Input: part model. Units: mm. Frame: model coordinates. A direction names the side the tool comes from. Coordinates: 2 decimals unless noted, no trailing zeros. Loops run counter-clockwise (first coordinate to the right, second up) from the corner with the lowest first, then second, coordinate; pieces in that order, holes last.
Item 1: Contact query for flat-ended pins moving along their axis: P1, Ø12, axis at x = -10.5, z = 0.5, coming from the -Y side; P2, Ø3, axis at x = -42.5, z = 0, coming from the +Y side; P3, Ø3, axis at x = 11.5, z = -12, coming from the +Y side. Output: stop coordinate, or through.
Item 2: Section B-B on y = 0.45. Return loops of the section in (x, z).
Item 3: Pull-direction query (Z, two-part tool) for faces 3 (the cylindrical face through (-47.01, 0.79, 0.1)), 4 (the cylindrical face through (-1.673, 1.354, -0.074)), 5 (the cylindrical face through (-35.32, 0.79, -9.96)); classes: released by +Z, released by -Z, zero draft, split by the parting line, or undercut.
Item 4: Section C-C on x = -0.5. Return loops of the section in (y, z), and give its area (3 significant figures).
Item 5: Ray query, line 1 along Z through (x, y) = (0, 1.4) (3 decimals); line 2 along X through (y, z) = (1.4, -38.1); line 3 along Z through (x, y) = (-42.5, 1.05). Return the intervals inside material, ascending.
Item 6: Reachability of faces 1 (the flat face through (-13, 1.1, 12)), 2 (the cylindrical face through (-40.502, 0.789, -0.088)) from +Z, -Z, +X, -X, +Y, -Y: full face, straight path, thin tool, end or side. Return the list, or none.
Item 7: Section D-D on z = 28. Return loops of the section in (x, y).
Item 8: Section A-A on z = 0. Return loops of the section in (x, y) (1 decimal).
Autodesk Inventor part; units mm, degrees
ref_plane "YZ Plane" through (0, 0, 0) normal (1, 0, 0) x (0, 1, 0)
ref_plane "XZ Plane" through (0, 0, 0) normal (0, 1, 0) x (-1, 0, 0)
ref_plane "XY Plane" through (0, 0, 0) normal (0, 0, 1) x (1, 0, 0)
sketch "Sketch1" plane through (0, 0, 0) normal (0, 1, 0) x (-1, 0, 0)
  circle A0 centre (42.5, 0) radius 2
  circle A1 centre (-21.25, 36.8061) radius 2
  circle A2 centre (-21.25, -36.8061) radius 2
  line L0 (-21.25, -36.8061) -> (0, 0) construction
  arc A3 (-25.1562, -34.5508) -> (-20.8492, -41.2987) centre (-21.25, -36.8061) ccw
  line L1 (-21.25, 36.8061) -> (0, 0) construction
  arc A4 (-17.3438, 39.0613) -> (-25.1562, 34.5508) centre (-21.25, 36.8061) ccw
  line L2 (0, 0) -> (42.5, 0) construction
  arc A5 (42.5, -4.5105) -> (42.5, 4.5105) centre (42.5, 0) ccw
  line L3 (-21.6508, -41.2987) -> (28.2014, -41.2987)
  line L4 (28.2014, -41.2987) -> (33.3458, -35.9407)
  line L5 (33.3458, -35.9407) -> (33.3458, -15.3261)
  line L6 (-25.1562, -34.5508) -> (-22.1167, -29.2863)
  line L7 (36.421, -4.5105) -> (42.5, -4.5105)
  line L8 (42.5, 0) -> (36.6992, 0)
  line L9 (4.5105, 0) -> (0, 0)
  line L10 (42.5, 4.5105) -> (36.421, 4.5105)
  line L11 (-25.1562, 34.5508) -> (-22.1167, 29.2863)
  line L12 (-14.3043, 33.7968) -> (-17.3438, 39.0613)
  arc A6 (-22.1167, 29.2863) -> (-22.1167, -29.2863) centre (0, 0) ccw
  arc A7 (33.3458, -15.3261) -> (36.421, -4.5105) centre (0, 0) ccw
  arc A8 (36.421, 4.5105) -> (-14.3043, 33.7968) centre (0, 0) ccw
  point P0 (-10.625, -18.403)
  point P1 (-10.625, 18.403)
  point P2 (21.25, 0)
  dimension "d1" = 4
  dimension "d2" = 42.5
  dimension "d5" = 360
extrude "Extrusion1" add sketch "Sketch1" along normal blind 1.6 contours L6 A6 L11 A4 L12 A8 L10 A5 L7 A7 L5 L4 L3 A3
sketch "Sketch2" plane through (0, 1.6, 0) normal (0, 1, 0) x (1, 0, 0)
  line L0 (35, 0) -> (0, 0) construction
  circle A0 centre (12.5, 12.5) radius 3
  circle A1 centre (-12.5, 12.5) radius 3
  circle A2 centre (-12.5, -12.5) radius 3
  circle A3 centre (12.5, -12.5) radius 3
  line L1 (1.675, -1.675) -> (-1.675, -1.675)
  line L2 (-1.675, -1.675) -> (-1.675, 1.675)
  line L3 (-1.675, 1.675) -> (1.675, 1.675)
  line L4 (1.675, 1.675) -> (1.675, -1.675)
  line L5 (1.675, -1.675) -> (-1.675, 1.675) construction
  line L6 (-1.675, -1.675) -> (1.675, 1.675) construction
  circle A4 centre (0, 0) radius 1.675
  circle A5 centre (0, -28) radius 3.75
  line L7 (0, -28) -> (0, 0) construction
  line L8 (-42.5, -4.5105) -> (-36.421, -4.5105)
  arc A6 (-42.5, 4.5105) -> (-42.5, -4.5105) centre (-42.5, 0) ccw
  line L9 (-36.421, 4.5105) -> (-42.5, 4.5105)
  arc A7 (-33.3458, 15.3261) -> (-36.421, 4.5105) centre (0, 0) ccw
  line L10 (-33.3458, 35.9407) -> (-33.3458, 15.3261)
  line L11 (-28.2014, 41.2987) -> (-33.3458, 35.9407)
  line L12 (21.6508, 41.2987) -> (-28.2014, 41.2987)
  arc A8 (25.1562, 34.5508) -> (21.6508, 41.2987) centre (21.25, 36.8061) ccw
  line L13 (22.1167, 29.2863) -> (25.1562, 34.5508)
  arc A9 (22.1167, -29.2863) -> (22.1167, 29.2863) centre (0, 0) ccw
  line L14 (25.1562, -34.5508) -> (22.1167, -29.2863)
  arc A10 (17.3438, -39.0613) -> (25.1562, -34.5508) centre (21.25, -36.8061) ccw
  line L15 (14.3043, -33.7968) -> (17.3438, -39.0613)
  arc A11 (-36.421, -4.5105) -> (14.3043, -33.7968) centre (0, 0) ccw
  circle A12 centre (21.25, 36.8061) radius 2
  circle A13 centre (21.25, -36.8061) radius 2
  circle A14 centre (-42.5, 0) radius 2
  circle A15 centre (11, 38.1) radius 0.381
  circle A16 centre (14.4, 38.1) radius 0.381
  line L16 (11, 38.1) -> (14.4, 38.1) construction
  dimension "d23" = 35
  dimension "d24" = 360
  dimension "d25" = 12.5
  dimension "d26" = 12.5
  dimension "d27" = 6
  dimension "d28" = 360
  dimension "d31" = 3.35
  dimension "d32" = 28
  dimension "d33" = 7.5
  dimension "d34" = 11
  dimension "d36" = 38.1
  dimension "d37" = 3.4
  dimension "d38" = 0.762
extrude "Extrusion2" cut sketch "Sketch2" against normal blind 0.5 contours A0 | A1 | A2 | A3 | A4 | A5 | A15 | A16
properties part number "PCB"
Results found:
1. P1: stops at y = 0
1. P2: passes through
1. P3: stops at y = 1.1
2. outline: (-42.5, -4.51) - (-36.42, -4.51) arc R36.7 ccw to (-33.35, -15.33) - (-33.35, -35.94) - (-28.2, -41.3) - (21.65, -41.3) arc R4.51 ccw to (25.16, -34.55) - (22.12, -29.29) arc R36.7 ccw to (22.12, 29.29) - (25.16, 34.55) arc R4.51 ccw to (17.34, 39.06) - (14.3, 33.8) arc R36.7 ccw to (-36.42, 4.51) - (-42.5, 4.51) arc R4.51 ccw to start; hole circle Ø4 at (-42.5, 0); hole circle Ø4 at (21.25, -36.81); hole circle Ø4 at (21.25, 36.81)
3. face 3: split by the parting line
3. face 4: undercut
3. face 5: released by -Z
4. outline: (0, -41.3) - (1.6, -41.3) - (1.6, -1.6) - (1.1, -1.6) - (1.1, 1.6) - (1.6, 1.6) - (1.6, 24.28) - (1.1, 24.28) - (1.1, 31.72) - (1.6, 31.72) - (1.6, 36.7) - (0, 36.7) - close
4. area: 119 mm2
5. line 1: z = -41.299 to -1.675, 1.675 to 24.25, 31.75 to 36.699
5. line 2: x = -31.27 to 10.62, 11.38 to 14.02, 14.78 to 19.72, 22.78 to 25.57
5. line 3: z = -4.51 to -2, 2 to 4.51
6. face 1: +Y
6. face 2: +Y, -Y
7. outline: (-23.72, 0) - (23.72, 0) - (23.72, 1.6) - (3.75, 1.6) - (3.75, 1.1) - (-3.75, 1.1) - (-3.75, 1.6) - (-23.72, 1.6) - close
8. outline: (-47, 0) - (-44.5, 0) - (-44.5, 1.6) - (-47, 1.6) - close; (-40.5, 0) - (36.7, 0) - (36.7, 1.6) - (1.7, 1.6) - (1.7, 1.1) - (-1.7, 1.1) - (-1.7, 1.6) - (-40.5, 1.6) - close
